from build123d import *

# Parameters (mm, degrees)
SKETCH1_R           = 10
BOSS_EXTRUDE1_DEPTH = 15
SKETCH2_R           = 3.4
CUT_EXTRUDE1_DEPTH  = 54
SKETCH3_R           = 4.25
CUT_EXTRUDE2_DEPTH  = 28
FILLET1_R           = 1.5


with BuildPart() as part:
    # Sketch1 → Boss-Extrude1 (new body)
    with BuildSketch(Plane.XY):
        with BuildLine():
            Line((0, 0), (0, 33))
            Line((0, 33), (66.33, 33))
            Line((66.33, 33), (66.33, 0))
            Line((66.33, 0), (50.665, 0))
            Line((50.665, 0), (50.665, -24.529))
            ThreePointArc((50.665, -24.529), (33.165, -42.029), (15.665, -24.529))
            Line((15.665, -24.529), (15.665, 0))
            Line((15.665, 0), (0, 0))
        make_face()
        with Locations((33.165, -24.529)):
            Circle(SKETCH1_R, mode=Mode.SUBTRACT)
    extrude(amount=BOSS_EXTRUDE1_DEPTH)

    # Sketch2 → Cut-Extrude1 (cut)
    with BuildSketch(Plane(origin=(0, 33, 0), x_dir=(1, 0, 0), z_dir=(0, 1, 0))):
        with Locations(Location((58.831, -7.5, 0), (0, 0, 270))):
            Circle(SKETCH2_R)
        with Locations(Location((7.499, -7.5, 0), (0, 0, 180))):
            Circle(SKETCH2_R)
    extrude(amount=-CUT_EXTRUDE1_DEPTH, mode=Mode.SUBTRACT)

    # Sketch3 → Cut-Extrude2 (cut)
    with BuildSketch(Plane(origin=(0, 33, 0), x_dir=(1, 0, 0), z_dir=(0, 1, 0))):
        with Locations(Location((33.165, -7.5, 0), (0, 0, 270))):
            Circle(SKETCH3_R)
    extrude(amount=-CUT_EXTRUDE2_DEPTH, mode=Mode.SUBTRACT)

    # Fillet1
    fillet1_edges = [part.edges().sort_by_distance(p)[0] for p in [
        (0, 0, 7.5),
        (66.33, 0, 7.5),
    ]]
    fillet(fillet1_edges, radius=FILLET1_R)


solid = part.part
Model file for the job. Use its own axes, mm. A direction names the side the tool comes from. Give positions to 0.01 mm unless a question says otherwise; leave off trailing zeros. Write each loop counter-clockwise with the first axis right and the second up, starting at its lowest first coordinate (ties: lowest second). Pieces come first, ordered by that corner, then holes. Notation, with made-up numbers: M 24,5 L 62,5 A11 ccw 62,21 Z; hole C 70.25,-29 d11. An arc over 180 degrees is marked long. One line per item, written item: value. Start each with the question number.
Q1. Probe probe 1 along X at (y, z) = (17, 5.25); probe 2 along X at (y, z) = (2.5, 5); probe 3 along X at (y, z) = (17, 8.75). List the from-to ranges inside material, lowest first. Write a range as [from, to].
Q2. Two-plate mould, pull along Y, no slides. Class faces 1 (the cylindrical face through (33.55, -42.025, 7.395)), 2 (the flat face through (50.665, -12, 7)), 3 (the cylindrical face through (25.795, -17.771, 7.395)): +Y half, -Y half, draft (parallel to the pull), parting line (faces both ways), or undercut.
Q3. 3-axis set-ups, long thin cutter, end or side, ignore diameter. For faces 4 (the flat face through (55, 0, 7)), 5 (the cylindrical face through (4.358, 16.731, 6.198)), 6 (the flat face through (33, 5, 7)), 7 (the flat face through (15.665, -12, 7)): which of +Z, -Z, +X, -X, +Y, -Y reach the whole face in a straight line?
Q4. Drop flat-ended pins along their axis: pin 1 Ø6 at (x, z) = (46, 12) entering from -Y; pin 2 Ø5 at (y, z) = (-33, 12.5) entering from +X; pin 3 Ø4.5 at (y, z) = (-16, 4.5) entering from +X (3 decimals). Give the stop position or say it passes through.
Q5. Saw through at C-C, the plane x = 7.5. Write the cut outline in (y, z), plus the area to 3 significant figures.
Q6. Saw through at A-A, the plane z = 7.5. Write the cut outline in (x, y) (3 decimals).
Q7. Saw through at D-D, the plane y = -28.5. Write the cut outline in (x, z).
Q8. Saw through at B-B, the plane z = 13.75. Write the cut outline in (x, y) (3 decimals).
Output values:
1. probe 1: x = [0, 4.95], [10.05, 29.56], [36.77, 56.28], [61.38, 66.33]
1. probe 2: x = [0, 5.19], [9.8, 56.53], [61.14, 66.33]
1. probe 3: x = [0, 4.34], [10.66, 29.1], [37.23, 55.67], [61.99, 66.33]
2. face 1: -Y half
2. face 2: draft
2. face 3: undercut
3. face 4: +Z, -Z, +X, -Y
3. face 5: +Y, -Y
3. face 6: +Y
3. face 7: +Z, -Z, -X, -Y
4. pin 1: stops at y = -39
4. pin 2: stops at x = 49.61
4. pin 3: stops at x = 50.665
5. outline: M 0,0 L 33,0 L 33,4.1 L 0,4.1 Z; M 0,10.9 L 33,10.9 L 33,15 L 0,15 Z
5. area: 271 mm²
6. outline: M 0,1.5 A1.5 ccw 1.5,0 L 4.099,0 L 4.099,33 L 0,33 Z; M 10.899,0 L 15.665,0 L 15.665,-24.529 A17.5 ccw 50.665,-24.529 L 50.665,0 L 55.431,0 L 55.431,33 L 37.415,33 L 37.415,5 L 28.915,5 L 28.915,33 L 10.899,33 Z; M 62.231,0 L 64.83,0 A1.5 ccw 66.33,1.5 L 66.33,33 L 62.231,33 Z; hole C 33.165,-24.529 d20
7. outline: M 16.12,0 L 23.99,0 L 23.99,15 L 16.12,15 Z; M 42.34,0 L 50.21,0 L 50.21,15 L 42.34,15 Z
8. outline: M 0,1.5 A1.5 ccw 1.5,0 L 15.665,0 L 15.665,-24.529 A17.5 ccw 50.665,-24.529 L 50.665,0 L 64.83,0 A1.5 ccw 66.33,1.5 L 66.33,33 L 0,33 Z; hole C 33.165,-24.529 d20
